Verification items for the finished model (mm, model axes). A direction names the side the tool comes from. Round coordinates to 2 decimals unless told otherwise and drop trailing zeros. Loops run counter-clockwise (first coordinate to the right, second up) from the corner with the lowest first, then second, coordinate; pieces in that order, holes last. Notation, with made-up numbers: (67.25, 0) -> (113.25, 0) arc R19 cw to (113.25, 35) -> close; hole circle Ø5 at (33.25, -11). An arc over 180 degrees is marked (long way). Use CSV: the item, a comma, the result in double quotes. Start each with the question number.
```python
from build123d import *

# Parameters (mm, degrees)
EXTRUDE_1_DEPTH = 25
EXTRUDE_START   = 3
SKETCH_1_3_R    = 2
EXTRUDE_2_DEPTH = 4
EXTRUDE_START_2 = 20
EXTRUDE_3_DEPTH = 4


with BuildPart() as part:
    # Sketch 1 → Extrude 1 (new body)
    with BuildSketch(Plane.XY):
        with BuildLine():
            ThreePointArc((4.949747468, -0.707106781), (3.535533906, -3.535533906), (0.707106781, -4.949747468))
            Line((0.707106781, -4.949747468), (2.73923518, -6.981875867))
            ThreePointArc((2.73923518, -6.981875867), (5.303300859, -5.303300859), (6.981875867, -2.73923518))
            Line((6.981875867, -2.73923518), (4.949747468, -0.707106781))
        make_face()
        with BuildLine():
            Line((3.5, 6.633249581), (3.5, 3.570714214))
            ThreePointArc((3.5, 3.570714214), (4.609772229, 1.936491673), (5, 0))
            ThreePointArc((5, 0), (4.987421044, -0.3544451), (4.949747468, -0.707106781))
            Line((4.949747468, -0.707106781), (6.981875867, -2.73923518))
            ThreePointArc((6.981875867, -2.73923518), (7.369330669, -1.393902973), (7.5, 0))
            ThreePointArc((7.5, 0), (6.422616289, 3.872983346), (3.5, 6.633249581))
        make_face()
        with BuildLine():
            ThreePointArc((0.707106781, -4.949747468), (-4.483261085, -2.213677945), (-3.5, 3.570714214))
            Line((-3.5, 3.570714214), (-3.5, 6.633249581))
            ThreePointArc((-3.5, 6.633249581), (-6.818181651, -3.124483794), (2.73923518, -6.981875867))
            Line((2.73923518, -6.981875867), (0.707106781, -4.949747468))
        make_face()
        with BuildLine():
            Line((-3.5, 6.633249581), (-3.5, 3.570714214))
            ThreePointArc((-3.5, 3.570714214), (0, 5), (3.5, 3.570714214))
            Line((3.5, 3.570714214), (3.5, 6.633249581))
            ThreePointArc((3.5, 6.633249581), (0, 7.5), (-3.5, 6.633249581))
        make_face()
    extrude(amount=EXTRUDE_1_DEPTH)

    # Sketch 1_3 → Extrude 2 (add)
    with BuildSketch(Plane.XY.offset(EXTRUDE_START)):
        with BuildLine():
            Line((-3.5, 14), (-3.5, 6.633249581))
            ThreePointArc((-3.5, 6.633249581), (0, 7.5), (3.5, 6.633249581))
            Line((3.5, 6.633249581), (3.5, 14))
            ThreePointArc((3.5, 14), (0, 17.5), (-3.5, 14))
        make_face()
        with Locations((0, 14)):
            Circle(SKETCH_1_3_R, mode=Mode.SUBTRACT)
    extrude(amount=EXTRUDE_2_DEPTH)

    # Sketch 1_4 → Extrude 3 (add)
    with BuildSketch(Plane.XY.offset(EXTRUDE_START_2)):
        with BuildLine():
            ThreePointArc((6.981875867, -2.73923518), (5.303300859, -5.303300859), (2.73923518, -6.981875867))
            Line((2.73923518, -6.981875867), (9.899494937, -14.142135624))
            ThreePointArc((9.899494937, -14.142135624), (14.142135624, -14.142135624), (14.142135624, -9.899494937))
            Line((14.142135624, -9.899494937), (6.981875867, -2.73923518))
        make_face()
        with BuildLine():
            ThreePointArc((13.081475452, -10.960155108), (13.081475452, -13.081475452), (10.960155108, -13.081475452))
            Line((10.960155108, -13.081475452), (6.717514421, -8.838834765))
            ThreePointArc((6.717514421, -8.838834765), (6.717514421, -6.717514421), (8.838834765, -6.717514421))
            Line((8.838834765, -6.717514421), (13.081475452, -10.960155108))
        make_face(mode=Mode.SUBTRACT)
    extrude(amount=EXTRUDE_3_DEPTH)


solid = part.part
```
Q1. Cross-section at D-D (y = 2.5). Record the boundary of the cut face in (x, z), and give its area (3 significant figures).
Q2. Cross-section at B-B (z = 22.25). Record the boundary of the cut face in (x, y), and give its area (3 significant figures).
Q3. Cross-section at A-A (x = 0). Record the boundary of the cut face in (y, z), and give its area (3 significant figures).
Q4. Cross-section at C-C (z = 7.5). Record the boundary of the cut face in (x, y).
Q5. Depth check by flat-ended pin: pin 1 Ø5 at (y, z) = (-11.5, 15.5) entering from +X; pin 2 Ø5.5 at (x, y) = (0, 14) entering from +Z; pin 3 Ø3 at (y, z) = (10.5, 4) entering from -X; pin 4 Ø4 at (x, z) = (5, 11.5) entering from -Y. Enter the tip coordinate at first touch or a pass-through.
Q6. Tool access check on faces 4 (the face through (8.87, -10.99, 21.97)), 5 (the face through (2, -5, 0)), 6 (the face through (7, -10, 20)), 7 (the face through (-3.5, 10, 5)), 8 (the face through (3.5, 10, 5)). Record the directions out of +Z, -Z, +X, -X, +Y, -Y that give a thin tool (end or side, any length) a straight path to the whole face; none if there is none.
Q7. Release check for a two-part mould opening along X. For faces 1 (the face through (10.93, -8.81, 21.97)), 2 (the face through (7, -10, 24)), 3 (the face through (14.095, -14.188, 21.972)) record: +X half, -X half, draft (parallel to the pull), parting line (faces both ways), or undercut.
Q8. Thickness scan on L1, parallel to Z at x = 9, y = -6.5; L2, parallel to Z at x = 3.25, y = 12.5; L3, parallel to Y at x = 2.75, z = 15.25. Record the ranges inside material, lowest first. Write a range as from..to.
Answer list:
1,outline,"(-7.07, 0) -> (-4.33, 0) -> (-4.33, 25) -> (-7.07, 25) -> close; (4.33, 0) -> (7.07, 0) -> (7.07, 25) -> (4.33, 25) -> close"
1,area,"137 mm2"
2,outline,"(2.74, -6.98) -> (9.9, -14.14) arc R3 ccw to (14.14, -9.9) -> (6.98, -2.74) arc R7.5 ccw (long way) to start; hole circle Ø10 at (0, 0); hole (6.72, -8.84) -> (10.96, -13.08) arc R1.5 ccw to (13.08, -10.96) -> (8.84, -6.72) arc R1.5 ccw to start"
2,area,"145 mm2"
3,outline,"(-7.5, 0) -> (-5, 0) -> (-5, 25) -> (-7.5, 25) -> close; (5, 0) -> (7.5, 0) -> (7.5, 3) -> (12, 3) -> (12, 7) -> (7.5, 7) -> (7.5, 25) -> (5, 25) -> close; (16, 3) -> (17.5, 3) -> (17.5, 7) -> (16, 7) -> close"
3,area,"149 mm2"
4,outline,"circle Ø15 at (0, 0); hole circle Ø10 at (0, 0)"
5,pin 1,"passes through"
5,pin 2,"stops at z = 7"
5,pin 3,"stops at x = -3.5"
5,pin 4,"stops at y = -6.87"
6,face 4,"+Z, -Z"
6,face 5,"-Z, +X, -X, +Y, -Y"
6,face 6,"-Z, +X, -Y"
6,face 7,"+Z, -Z, -X, +Y"
6,face 8,"+Z, -Z, +X, +Y"
7,face 1,"undercut"
7,face 2,"draft"
7,face 3,"parting line"
8,L1,"z = 20..24"
8,L2,"z = 3..7"
8,L3,"y = -6.98..-4.18, 4.18..6.98"
